```python
from build123d import *

# Parameters (mm, degrees)
SKETCH1_R               = 12.5
BOSS_EXTRUDE1_DEPTH     = 3.3
CUT_EXTRUDE1_START      = -6.6
CUT_EXTRUDE1_DEPTH      = 26.469552194
CIRPATTERN2_COUNT       = 39
SKETCH2_R               = 15
BOSS_EXTRUDE3_DEPTH     = 1.5
BOSS_EXTRUDE4_START     = 1.5
SKETCH3_R               = 14.999999972
BOSS_EXTRUDE4_DEPTH     = 1.5
CUT_EXTRUDE3_DEPTH      = 24.284329494
CUT_EXTRUDE3_DEPTH_BACK = 24.284329494


with BuildPart() as part:
    # Sketch1 → Boss-Extrude1 (new, symmetric)
    with BuildSketch(Plane.XY):
        Circle(SKETCH1_R)
    extrude(amount=BOSS_EXTRUDE1_DEPTH, both=True)

    # Sketch4 → Cut-Extrude1 (cut)
    with BuildSketch(Plane.XY.offset(3.3).offset(CUT_EXTRUDE1_START)):
        Polygon((-0.6, 11.75), (0.6, 11.75), (0.8, 12.5), (-0.8, 12.5), align=None)
    cut_extrude1 = extrude(amount=CUT_EXTRUDE1_DEPTH, mode=Mode.SUBTRACT)

    # CirPattern2: Cut-Extrude1 ×39 about axis
    cirpattern2_axis = Axis((0, 0, 0), (0, 0, 1))
    for i in range(1, CIRPATTERN2_COUNT):
        add(cut_extrude1.rotate(cirpattern2_axis, i * 360 / CIRPATTERN2_COUNT), mode=Mode.SUBTRACT)

    # Sketch2 → Boss-Extrude3 (add)
    with BuildSketch(Plane(origin=(0, 0, -3.3), x_dir=(-1, 0, 0), z_dir=(0, 0, -1))):
        Circle(SKETCH2_R)
    extrude(amount=BOSS_EXTRUDE3_DEPTH)

    # Sketch3 → Boss-Extrude4 (add)
    with BuildSketch(Plane.XY.offset(3.3).offset(BOSS_EXTRUDE4_START)):
        with Locations(Location((0, 0, 0), (0, 0, 180))):
            Circle(SKETCH3_R)
    extrude(amount=-BOSS_EXTRUDE4_DEPTH)

    # Sketch6 → Cut-Extrude3 (cut, two sides: drawn at the far end of the back side and taken through both)
    with BuildSketch(Plane.XY.offset(4.8).offset(-CUT_EXTRUDE3_DEPTH_BACK)):
        with BuildLine():
            Line((5.303300859, 8.625), (-5.303300859, 8.625))
            ThreePointArc((-5.303300859, 8.625), (-4.940632743, -8.83774706), (10.125, 0))
            ThreePointArc((10.125, 0), (8.83774706, 4.940632743), (5.303300859, 8.625))
        make_face()
    extrude(amount=CUT_EXTRUDE3_DEPTH + CUT_EXTRUDE3_DEPTH_BACK, mode=Mode.SUBTRACT)


solid = part.part
```
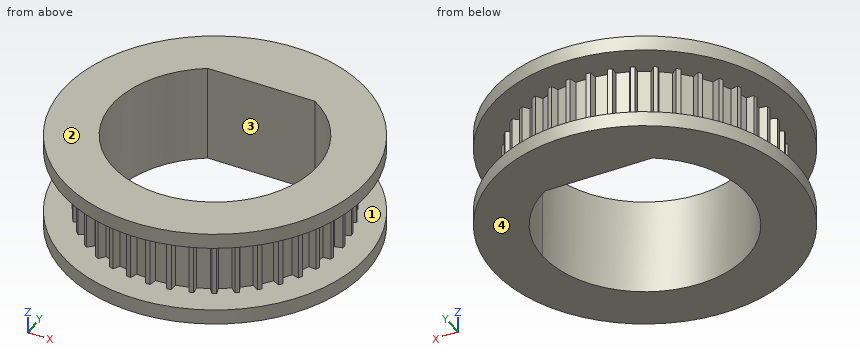
The model under review builds one solid part; all positions refer to its coordinate system, in mm. Face numbers are marked on the shaded views. A direction names the side the tool comes from. Give positions to 0.01 mm unless a question says otherwise; leave off trailing zeros. Loops run counter-clockwise (first coordinate to the right, second up) from the corner with the lowest first, then second, coordinate; pieces in that order, holes last. Notation, with made-up numbers: (14.5, -28) - (47.5, -28) arc R29 cw to (47.5, -6) - close; hole circle Ø5 at (41, 54.25). An arc over 180 degrees is marked (long way). Answer as a JSON object with one key per item and string values.
Q1. Mouldability with a two-part tool opening along Y and no side actions: class the marked faces 3 and 4 as +Y half, -Y half, draft (parallel to the pull), parting line (faces both ways), or undercut.
Worked out:
{"face 3": "undercut", "face 4": "draft"}
Q2. Add section A-A on y = 5. State the section outline as (x, z) points.
Worked out:
{"outline": "(-14.14, -4.8) - (-8.8, -4.8) - (-8.8, 4.8) - (-14.14, 4.8) - (-14.14, 3.3) - (-10.63, 3.3) - (-10.63, -3.3) - (-14.14, -3.3) - close; (8.8, -4.8) - (14.14, -4.8) - (14.14, -3.3) - (10.63, -3.3) - (10.63, 3.3) - (14.14, 3.3) - (14.14, 4.8) - (8.8, 4.8) - close"}
Q3. For the marked faces 1 and 2, list the 3-axis set-ups (+Z, -Z, +X, -X, +Y, -Y) from which the entire face can be reached by the end or side of a thin tool; tool diameter is ignored.
Worked out:
{"face 1": "none", "face 2": "+Z, +X, -X, +Y, -Y"}
Q4. To check wall thickness, follow line 1 along Z through (x, y) = (-11.5, 9.5); line 2 along Y through (x, z) = (0, -0.75) (3 decimals); line 3 along Y through (x, z) = (-7.5, 1.5). State the ranges of each line that lie inside material, in increasing order.
Worked out:
{"line 1": "z = -4.8 to -3.3, 3.3 to 4.8", "line 2": "y = -12.5 to -10.125, 8.625 to 11.75", "line 3": "y = -10 to -9.51, -9.05 to -6.8, 6.8 to 9.06"}
Q5. Add section B-B on z = 3.75. State the section outline as (x, y) points (3 decimals).
Worked out:
{"outline": "circle Ø30 at (0, 0); hole (-5.303, 8.625) arc R10.125 ccw (long way) to (5.303, 8.625) - close"}
Q6. Insertion check: pin 1 (5 mm diameter, centred on y = 9.5, z = 3, fed in from -X); pin 2 (3 mm diameter, centred on x = -1, z = 1.5, fed in from -Y); pin 3 (2 mm diameter, centred on y = 7.5, z = -3, fed in from -X); pin 4 (16 mm diameter, centred on x = 0, y = 0, fed in from -Z). Each pin has a flat end and moves straight along its axis. Give the tip position at first contact, or say it passes through.
Worked out:
{"pin 1": "stops at x = -13.26", "pin 2": "stops at y = -12.5", "pin 3": "stops at x = -13.5", "pin 4": "passes through"}
